Autodesk Inventor part; units mm, degrees
ref_plane "Work Plane1" through (-3, -2.69, 0) normal (0, 1, 0) x (1, 0, 0)
ref_plane "YZ Plane" through (0, 0, 0) normal (1, 0, 0) x (0, 1, 0)
ref_plane "XZ Plane" through (0, 0, 0) normal (0, 1, 0) x (-1, 0, 0)
sketch "Sketch1" plane through (0, 0, 0) normal (0, 0, 1) x (1, 0, 0)
  circle A0 centre (0, 0) radius 1
  line L0 (-8.2702, 3.81) -> (10.8086, 3.81) construction
  arc A1 (-2.4804, -0.3126) -> (2.4804, -0.3126) centre (0, 0) ccw
  line L1 (0, 0) -> (2.4804, -0.3126) construction
  line L2 (-3, 3.81) -> (-3, 5.81)
  line L3 (-3, 5.81) -> (3, 5.81)
  line L4 (3, 5.81) -> (3, 3.81)
  line L5 (0, 5.81) -> (0, -5.1474) construction
  line L6 (2.4804, -0.3126) -> (3, 3.81)
  line L7 (-2.4804, -0.3126) -> (-3, 3.81)
  dimension "d0" = 2
  dimension "d3" = 3.81
  dimension "d4" = 2
  dimension "d5" = 6
  dimension "d6" = 2.5
extrude "Extrusion1" add sketch "Sketch1" along normal blind 5
sketch "Sketch2" plane through (3, 3.81, 0) normal (1, 0, 0) x (0, 0, -1)
  line L0 (-5, 0) -> (-5, 2)
  line L1 (0, 0) -> (-5, 0)
  line L2 (-4, 0) -> (-3, 0)
  line L3 (-3, 0) -> (-3, -8)
  line L4 (-3, -8) -> (-4, -8)
  line L5 (-4, -8) -> (-4, 0)
  point P0 (0, -3.81)
  dimension "d7" = 1
  dimension "d9" = 1
  dimension "d10" = 8
extrude "Extrusion2" cut sketch "Sketch2" against normal blind 10
sketch "Sketch3" plane through (0, 0, 3) normal (0, 0, 1) x (1, 0, 0)
  arc A0 (-2.4804, -0.3126) -> (2.4804, -0.3126) centre (0, 0) ccw
  line L0 (3, 3.81) -> (-3, 3.81)
  circle A1 centre (0, 0) radius 1
  line L1 (0, 2.3094) -> (2, 1.1547)
  line L2 (2, 1.1547) -> (2, -1.1547)
  line L3 (2, -1.1547) -> (0, -2.3094)
  line L4 (0, -2.3094) -> (-2, -1.1547)
  line L5 (-2, -1.1547) -> (-2, 1.1547)
  line L6 (-2, 1.1547) -> (0, 2.3094)
  line L7 (0, 3.81) -> (0, 1.7188) construction
  point P0 (0, 0)
  dimension "d13" = 2
extrude "Extrusion3" cut sketch "Sketch3" against normal blind 2.5
sketch "Sketch5" plane through (0, 0, 3) normal (0, 0, 1) x (1, 0, 0)
  line L0 (-2, 1.1547) -> (0, 2.3094)
  line L1 (0, 2.3094) -> (2, 1.1547)
  line L2 (2, 1.1547) -> (2, -1.1547)
  line L3 (2, -1.1547) -> (0, -2.3094)
  line L4 (0, -2.3094) -> (-2, -1.1547)
  line L5 (-2, -1.1547) -> (-2, 1.1547)
  circle A0 centre (0, 0) radius 1
extrude "Extrusion5" add sketch "Sketch5" against normal blind 0.5
ref_plane "Work Plane1" through (-3, -2.69, 0) normal (0, 1, 0) x (1, 0, 0)
sketch "Sketch6" plane through (-3, -2.69, 0) normal (0, 1, 0) x (1, 0, 0)
  line L0 (1, -2.5) -> (3, -2.5)
  line L1 (3, -2.5) -> (3, -0.5)
  line L2 (1, -2.5) -> (1, -0.5)
  line L3 (3, -2.5) -> (5, -2.5)
  line L4 (5, -2.5) -> (5, -0.5)
  line L5 (3, -2.5) -> (3, -0.5)
  line L6 (4.9, -0.6) -> (1.1, -0.6)
  line L7 (1.1, -0.6) -> (1.1, -2.4)
  line L8 (1.1, -2.4) -> (4.9, -2.4)
  line L9 (4.9, -2.4) -> (4.9, -0.6)
  line L10 (5, -0.5) -> (3, -0.5)
  line L11 (3, -0.5) -> (1, -0.5)
  point P0 (3, 0)
  dimension "d28" = 0.1
  dimension "d29" = 0.1
  dimension "d30" = 0.1
extrude "Extrusion6" cut sketch "Sketch6" along normal blind 2 and the other way blind 2 contours L8 L7 L6 L1 | L1 L6 L9 L8
sketch "Sketch7" plane through (0, 0, 5) normal (0, 0, 1) x (1, 0, 0)
  circle A0 centre (0, 0) radius 1
  arc A1 (-2.4804, -0.3126) -> (2.4804, -0.3126) centre (0, 0) ccw
  line L0 (2.4804, -0.3126) -> (3, 3.81)
  line L1 (3, 3.81) -> (3, 5.21)
  line L2 (2.4, 5.81) -> (-2.4, 5.81)
  line L3 (-3, 5.21) -> (-3, 3.81)
  line L4 (-3, 3.81) -> (-2.4804, -0.3126)
  line L5 (-3, 3.81) -> (3, 3.81)
  arc A2 (-2.4, 5.81) -> (-3, 5.21) centre (-2.4, 5.21) ccw
  arc A3 (3, 5.21) -> (2.4, 5.81) centre (2.4, 5.21) ccw
  line L6 (2.4804, -0.3126) -> (3, 3.81)
  line L7 (-3, 5.81) -> (-3, 3.81)
  line L8 (-3, 3.81) -> (-2.4804, -0.3126)
  line L9 (-2.7479, 1.81) -> (2.7479, 1.81)
  dimension "d35" = 2
fillet "Fillet1" radius 0.6 2 edges at (3, 5.81, 2.5) (-3, 5.81, 2.5)
extrude "Extrusion7" cut sketch "Sketch7" against normal blind 2 contours L4 L9 L0 A1
sketch "Sketch8" plane through (0, 0, 3) normal (0, 0, 1) x (1, 0, 0)
  circle A0 centre (0, 0) radius 1
  arc A1 (-2.4804, -0.3126) -> (2.4804, -0.3126) centre (0, 0) ccw
  circle A2 centre (0, 0) radius 1.4
  circle A3 centre (0, 0) radius 1
  dimension "d36" = 2.8
  dimension "d37" = 2
extrude "Extrusion8" add sketch "Sketch8" along normal blind 0.5
properties part number "HexSaver01"
Here's how the part is built. I have some questions about the finished solid (model axes, mm). A direction names the side the tool comes from. Coordinates: 2 decimals unless noted, no trailing zeros. Loops run counter-clockwise (first coordinate to the right, second up) from the corner with the lowest first, then second, coordinate; pieces in that order, holes last. Notation, with made-up numbers: (-40, -6) - (-6, -6) arc R23 ccw to (-6, 16) - close; hole circle Ø9 at (-1.5, -24). An arc over 180 degrees is marked (long way). Return JSON: item names as keys, results as strings. Group by question number.
Item 1: I need wall thicknesses on line 1 (Z direction, x = -1, y = 3.5); line 2 (Y direction, x = 0, z = 0.2); line 3 (Z direction, x = 1.75, y = 0.75). Which ranges of each line are inside material? Lowest first, please. Write a range as from..to.
Item 2: On a 3-axis mill with a long thin cutter (end or side, diameter ignored), from which of +Z, -Z, +X, -X, +Y, -Y can I reach the whole of each face in a straight line? I mean faces 1 (the face through (2, 0, 2)), 2 (the face through (0, 3.81, 3.5)), 3 (the face through (-0.4, -2.3, 0.6)). Say none if no direction works.
Item 3: If we section it at C-C on x = 0.5: Write out the boundary of the cut face in (y, z), and give its area (3 significant figures).
Item 4: If we section it at D-D on z = 1.55: Write out the boundary of the cut face in (x, y).
Item 5: We'd pull the mould along Z, two halves only. Please class faces 4 (the face through (-1, 1, 0.5)), 5 (the face through (3, 5, 2)), 6 (the face through (0, 3, 0)), 7 (the face through (0, 4, 5)): +Z half, -Z half, draft (parallel to the pull), parting line (faces both ways), or undercut.
Item 6: If we section it at A-A on z = 3.2: Write out the boundary of the cut face in (x, y), and give its area (3 significant figures).
Item 7: If we section it at B-B on y = 0: Write out the boundary of the cut face in (x, z), and give its area (3 significant figures).
Item 8: Will these pins go through, and if not, where does the flat tip stop? P1, Ø0.5, axis at y = -1.5, z = 1.5, coming from the +X side; P2, Ø2, axis at x = 2, y = -0.5, coming from the +Z side; P3, Ø1.5, axis at x = 2, z = 2, coming from the -Y side.
Calculated:
{
 "1": {"line 1": "z = 0..3, 4..5", "line 2": "y = -2.5..-1, 1..5.81", "line 3": "z = 0..0.5, 2.5..3"},
 "2": {"face 1": "none", "face 2": "+X, -X", "face 3": "-Y"},
 "3": {"outline": "(-2.45, 0) - (-0.87, 0) - (-0.87, 0.5) - (-2.02, 0.5) - (-2.02, 0.6) - (-2.45, 0.6) - close; (-2.45, 2.4) - (-2.02, 2.4) - (-2.02, 2.5) - (-0.87, 2.5) - (-0.87, 3.5) - (-1.31, 3.5) - (-1.31, 3) - (-2.45, 3) - close; (0.87, 0) - (5.81, 0) - (5.81, 5) - (1.81, 5) - (1.81, 4) - (3.81, 4) - (3.81, 3) - (1.31, 3) - (1.31, 3.5) - (0.87, 3.5) - (0.87, 2.5) - (2.02, 2.5) - (2.02, 0.5) - (0.87, 0.5) - close", "area": "20.6 mm^2"},
 "4": {"outline": "(-3, 3.81) - (-2.48, -0.31) arc R2.5 ccw to (-1.9, -1.62) - (-1.9, -1.21) - (-2, -1.15) - (-2, 1.15) - (0, 2.31) - (2, 1.15) - (2, -1.15) - (1.9, -1.21) - (1.9, -1.62) arc R2.5 ccw to (2.48, -0.31) - (3, 3.81) - (3, 5.21) arc R0.6 ccw to (2.4, 5.81) - (-2.4, 5.81) arc R0.6 ccw to (-3, 5.21) - close"},
 "5": {"face 4": "undercut", "face 5": "draft", "face 6": "-Z half", "face 7": "+Z half"},
 "6": {"outline": "(-3, 3.81) - (3, 3.81) - (3, 5.21) arc R0.6 ccw to (2.4, 5.81) - (-2.4, 5.81) arc R0.6 ccw to (-3, 5.21) - close; circle Ø2.8 at (0, 0); hole circle Ø2 at (0, 0)", "area": "14.9 mm^2"},
 "7": {"outline": "(-2.52, 0) - (-1, 0) - (-1, 0.5) - (-2, 0.5) - (-2, 2.5) - (-1, 2.5) - (-1, 3.5) - (-1.4, 3.5) - (-1.4, 3) - (-2.52, 3) - close; (1, 0) - (2.52, 0) - (2.52, 3) - (1.4, 3) - (1.4, 3.5) - (1, 3.5) - (1, 2.5) - (2, 2.5) - (2, 0.5) - (1, 0.5) - close", "area": "5.52 mm^2"},
 "8": {"P1": "stops at x = 2.17", "P2": "stops at z = 3.5", "P3": "stops at y = -2.09"}
}
